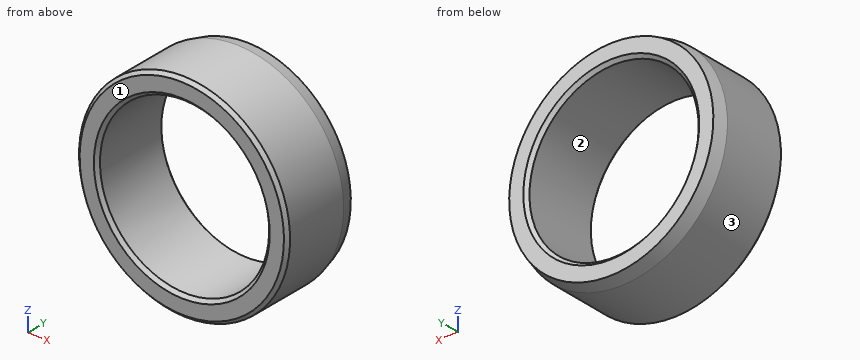
```python
from build123d import *

# Parameters (mm, degrees)
F0_W     = 24
F0_H     = 6.2484
F2_SIZE  = 1
F3_SIZE2 = 1.020886
F3_SIZE  = 3.81


with BuildPart() as f1:
    # F0 (on Right) → F1 (revolve)
    with BuildSketch(Plane.YZ):
        with Locations((12, 28.4099)):
            Rectangle(F0_W, F0_H)
    revolve(axis=Axis((0, 10.069529, 0), (0, 1, 0)))

    # F2
    f2_edges = [f1.edges().sort_by_distance(p)[0] for p in [
        (0, 0, -25.2857),
        (0, 0, -31.5341),
        (0, 24, -25.2857),
    ]]
    chamfer(f2_edges, length=F2_SIZE)

    # F3
    f3_edges = [f1.edges().sort_by_distance(p)[0] for p in [
        (0, 24, -31.5341),
    ]]
    chamfer(f3_edges, length=F3_SIZE, length2=F3_SIZE2)


solid = f1.part
```
Work out the finished part from the listing and answer in its coordinate system (mm). Face numbers are marked on the shaded views. Round coordinates to 2 decimals unless told otherwise and drop trailing zeros. Write each loop counter-clockwise with the first axis right and the second up, starting at its lowest first coordinate (ties: lowest second). Pieces come first, ordered by that corner, then holes.
1) Consider probe 1 along X at (y, z) = (16, 0); probe 2 along Z at (x, y) = (-12.5, 6); probe 3 along X at (y, z) = (21.75, 20). Determine where each line is inside the solid, lowest interval first.
2) A cutting plane is placed at C-C on y = 4.25. Determine the outline of the cut face in (x, z), and give its area (3 significant figures).
3) A cutting plane is placed at A-A on x = 0. Determine the outline of the cut face in (y, z).
4) Determine the mould class of the marked faces 1, 2 and 3 for opening direction Z: pulls with the +Z half, pulls with the -Z half, needs draft (parallel to the pull), parting line crosses it, or undercut.
5) Flat-ended cylindrical pins translate along their axes: P1, Ø12, axis at x = 12.5, y = 15.5, coming from the +Z side; P2, Ø1.5, axis at y = 7, z = 9, coming from the -X side; P3, Ø10, axis at x = -19, y = 7.5, coming from the -Z side; P4, Ø10, axis at x = 14, z = 9.5, coming from the -Y side. Find the tip coordinate at first contact, or state that the pin passes through.
6) A cutting plane is placed at B-B on z = 0. Determine the outline of the cut face in (x, y).
Entries:
1. probe 1: x = -31.53 to -25.29, 25.29 to 31.53
1. probe 2: z = -28.95 to -21.98, 21.98 to 28.95
1. probe 3: x = -23.84 to -15.47, 15.47 to 23.84
2. outline: circle Ø63.07 at (0, 0); hole circle Ø50.57 at (0, 0)
2. area: 1,120 mm2
3. outline: (0, -30.53) - (1, -31.53) - (20.19, -31.53) - (24, -30.51) - (24, -26.29) - (23, -25.29) - (1, -25.29) - (0, -26.29) - close; (0, 26.29) - (1, 25.29) - (23, 25.29) - (24, 26.29) - (24, 30.51) - (20.19, 31.53) - (1, 31.53) - (0, 30.53) - close
4. face 1: needs draft
4. face 2: undercut
4. face 3: parting line crosses it
5. P1: stops at z = 30.86
5. P2: stops at x = -30.44
5. P3: stops at z = -28.26
5. P4: passes through
6. outline: (-31.53, 1) - (-30.53, 0) - (-26.29, 0) - (-25.29, 1) - (-25.29, 23) - (-26.29, 24) - (-30.51, 24) - (-31.53, 20.19) - close; (25.29, 1) - (26.29, 0) - (30.53, 0) - (31.53, 1) - (31.53, 20.19) - (30.51, 24) - (26.29, 24) - (25.29, 23) - close
